```python
from build123d import *

# Parameters (mm, degrees)
F0_W      = 35
F0_H      = 35
F0_W_2    = 20
F0_H_2    = 20
F1_DEPTH  = 60
F3_R      = 2
F4_DEPTH  = 10
F6_W      = 35
F6_H      = 30
F6_W_2    = 20
F6_H_2    = 20
F7_DEPTH  = 50
F8_DEPTH  = 17.5
F9_DEPTH  = 60
F10_DEPTH = 10.25
F11_DEPTH = 55
F12_R     = 5
F13_R     = 2
F14_DEPTH = 20


# Not quite as in the source:
# - a feature of the source that left no trace in its solid (it failed there, or was rolled back) is left out


with BuildPart() as f1:
    # F0 (on Top) → F1 (new body)
    with BuildSketch(Plane.XY):
        Rectangle(F0_W, F0_H)
        Rectangle(F0_W_2, F0_H_2, mode=Mode.SUBTRACT)
    extrude(amount=F1_DEPTH)

    # F3 (on face) → F4 (cut)
    with BuildSketch(Plane.YZ.offset(17.5)):
        with Locations((0, 40)):
            Circle(F3_R)
        with Locations((0, 15)):
            Circle(F3_R)
    extrude(amount=-F4_DEPTH, mode=Mode.SUBTRACT)

    # F6 (on Right) → F7 (join)
    with BuildSketch(Plane.YZ):
        with Locations((0, 45)):
            Rectangle(F6_W, F6_H)
        with Locations((0, 45)):
            Rectangle(F6_W_2, F6_H_2, mode=Mode.SUBTRACT)
        with Locations((0, 45)):
            Rectangle(F6_W_2, F6_H_2)
    extrude(amount=F7_DEPTH)

    # F6 (on Right) → F8 (join, through all)
    with BuildSketch(Plane.YZ):
        with Locations((0, 45)):
            Rectangle(F6_W, F6_H)
        with Locations((0, 45)):
            Rectangle(F6_W_2, F6_H_2, mode=Mode.SUBTRACT)
        with Locations((0, 45)):
            Rectangle(F6_W_2, F6_H_2)
    extrude(amount=-F8_DEPTH)

    # F6 (on Right) → F9 (cut)
    with BuildSketch(Plane.YZ):
        with Locations((0, 45)):
            Rectangle(F6_W_2, F6_H_2)
    extrude(amount=F9_DEPTH, mode=Mode.SUBTRACT)

    # F6 (on Right) → F10 (cut)
    with BuildSketch(Plane.YZ):
        with Locations((0, 45)):
            Rectangle(F6_W_2, F6_H_2)
    extrude(amount=-F10_DEPTH, mode=Mode.SUBTRACT)

    # F0 (on Top) → F11 (cut, through all)
    with BuildSketch(Plane.XY):
        Rectangle(F0_W_2, F0_H_2)
    extrude(amount=F11_DEPTH, mode=Mode.SUBTRACT)

    # F12
    f12_edges = [f1.edges().sort_by_distance(p)[0] for p in [
        (-17.5, -17.5, 30),
        (-17.5, 17.5, 30),
        (33.75, -17.5, 30),
        (33.75, 17.5, 30),
        (16.25, 17.5, 60),
        (16.25, -17.5, 60),
        (17.5, -17.5, 15),
        (17.5, 17.5, 15),
    ]]
    fillet(f12_edges, radius=F12_R)

    # F13 (on face) → F14 (cut)
    with BuildSketch(Plane(origin=(0, 0, 30), x_dir=(1, 0, 0), z_dir=(0, 0, -1))):
        with Locations((35, 0)):
            Circle(F13_R)
    extrude(amount=-F14_DEPTH, mode=Mode.SUBTRACT)


solid = f1.part
```
Could you check a few things on this model? Use its own coordinates, in mm. A direction names the side the tool comes from. Round coordinates to 2 decimals unless told otherwise and drop trailing zeros. Order: outer loops, then holes, each group sorted by start corner. A loop starts at its lowest first (then second) coordinate and runs counter-clockwise, first axis right, second up. Notation, with made-up numbers: (46.5, 30.5) -> (52.5, 30.5) arc R25 ccw to (52.5, 48.5) -> close; hole circle Ø3 at (-15, 34). An arc over 180 degrees is marked (long way). One line per question, with ' | ' between items.
Q1. If we section it at C-C on x = 38: Write out the boundary of the cut face in (y, z), plus the area to 3 significant figures.
Computed values:
outline: (-17.5, 35) arc R5 ccw to (-12.5, 30) -> (12.5, 30) arc R5 ccw to (17.5, 35) -> (17.5, 55) arc R5 ccw to (12.5, 60) -> (-12.5, 60) arc R5 ccw to (-17.5, 55) -> close; hole (-10, 35) -> (10, 35) -> (10, 55) -> (-10, 55) -> close | area: 629 mm²
Q2. If I drill on line 1 (X direction, y = 0, z = 31); line 2 (Z direction, x = 13.5, y = 0); line 3 (X direction, y = -4, z = 19.5), over which ranges is the centre line in solid material (lowest first)? Write a range as from..to.
Computed values:
line 1: -17.5..-10, 10..33, 37..50 | line 2: 0..13, 17..35, 55..60 | line 3: -17.5..-10, 10..17.5
Q3. If we section it at D-D on z = 31: Write out the boundary of the cut face in (x, y), plus the area to 3 significant figures.
Computed values:
outline: (-17.5, -12.5) arc R5 ccw to (-12.5, -17.5) -> (12.5, -17.5) arc R5 ccw to (16.5, -15.5) -> (50, -15.5) -> (50, 15.5) -> (16.5, 15.5) arc R5 ccw to (12.5, 17.5) -> (-12.5, 17.5) arc R5 ccw to (-17.5, 12.5) -> close; hole (-10, -10) -> (10, -10) -> (10, 10) -> (-10, 10) -> close; hole circle Ø4 at (35, 0) | area: 1,800 mm²
Q4. If we section it at B-B on x = 11: Write out the boundary of the cut face in (y, z), plus the area to 3 significant figures.
Computed values:
outline: (-17.5, 0) -> (17.5, 0) -> (17.5, 55) arc R5 ccw to (12.5, 60) -> (-12.5, 60) arc R5 ccw to (-17.5, 55) -> close; hole (-10, 35) -> (10, 35) -> (10, 55) -> (-10, 55) -> close; hole circle Ø4 at (0, 15) | area: 1,680 mm²
Q5. We'd pull the mould along Z, two halves only. Please class faces 4 (the face through (30, 0, 35)), 5 (the face through (15.78, -16.07, 58.5)), 6 (the face through (31.51, 16.07, 31.5)), 7 (the face through (16, 16.07, 17.74)): released by +Z, released by -Z, zero draft, split by the parting line, or undercut.
Computed values:
face 4: undercut | face 5: released by +Z | face 6: released by -Z | face 7: zero draft
Q6. I'm going to push flat-ended pins straight in: pin 1 (10 mm diameter, centred on y = -13, z = 30, fed in from +X); pin 2 (12.5 mm diameter, centred on x = 36.5, y = 0, fed in from -Z); pin 3 (6 mm diameter, centred on y = 2, z = 47, fed in from +X); pin 4 (7.5 mm diameter, centred on y = 4, z = 17, fed in from +X). Where does each tip first touch, or does it pass through?
Computed values:
pin 1: x = 50 | pin 2: z = 30 | pin 3: x = -10.25 | pin 4: x = 17.5
Q7. If we section it at A-A on y = 0: Write out the boundary of the cut face in (x, z), plus the area to 3 significant figures.
Computed values:
outline: (-17.5, 0) -> (-10, 0) -> (-10, 35) -> (-10.25, 35) -> (-10.25, 55) -> (50, 55) -> (50, 60) -> (-17.5, 60) -> close; (10, 0) -> (17.5, 0) -> (17.5, 13) -> (10, 13) -> close; (10, 17) -> (17.5, 17) -> (17.5, 30) -> (33, 30) -> (33, 35) -> (10, 35) -> close; (37, 30) -> (50, 30) -> (50, 35) -> (37, 35) -> close | area: 1,120 mm²
Q8. Which directions (+Z, -Z, +X, -X, +Y, -Y) give clear straight access to the entire face, cutting with the end or side of a thin tool? Please do faces 1 (the face through (31.51, -16.07, 31.5)), 2 (the face through (13, 10, 39)), 3 (the face through (36.847, 0.766, 32.465)).
Computed values:
face 1: -Z, +X, -Y | face 2: none | face 3: -Z
